```python
from build123d import *

# Parameters (mm, degrees)
BOSS_EXTRUDE2_DEPTH = 2
BOSS_EXTRUDE3_DEPTH = 10.9


with BuildPart() as part:
    # Sketch1 → Boss-Extrude2 (new body)
    with BuildSketch(Plane(origin=(0, 0, 0), x_dir=(1, 0, 0), z_dir=(0, 1, 0))):
        with BuildLine():
            Line((0, 28.575), (137.052797764, 28.575))
            ThreePointArc((137.052797764, 28.575), (139.26125033, 14.36329198), (140, 0))
            ThreePointArc((140, 0), (139.26125033, -14.36329198), (137.052797764, -28.575))
            Line((137.052797764, -28.575), (0, -28.575))
            ThreePointArc((0, -28.575), (-28.575, 0), (0, 28.575))
        make_face()
    extrude(amount=-BOSS_EXTRUDE2_DEPTH)

    # Sketch1_14 → Boss-Extrude3 (add)
    with BuildSketch(Plane(origin=(0, 0, 0), x_dir=(1, 0, 0), z_dir=(0, 1, 0))):
        with BuildLine():
            Line((0, 28.575), (137.052797764, 28.575))
            ThreePointArc((137.052797764, 28.575), (139.26125033, 14.36329198), (140, 0))
            ThreePointArc((140, 0), (139.26125033, -14.36329198), (137.052797764, -28.575))
            Line((137.052797764, -28.575), (0, -28.575))
            ThreePointArc((0, -28.575), (-28.575, 0), (0, 28.575))
        make_face()
        with BuildLine():
            Line((0, -26.575), (130.828205579, -26.575))
            ThreePointArc((130.828205579, -26.575), (132.830371988, -13.354485299), (133.5, 0))
            ThreePointArc((133.5, 0), (132.830371988, 13.354485299), (130.828205579, 26.575))
            Line((130.828205579, 26.575), (0, 26.575))
            ThreePointArc((0, 26.575), (-26.575, 0), (0, -26.575))
        make_face(mode=Mode.SUBTRACT)
    extrude(amount=BOSS_EXTRUDE3_DEPTH)


solid = part.part
```
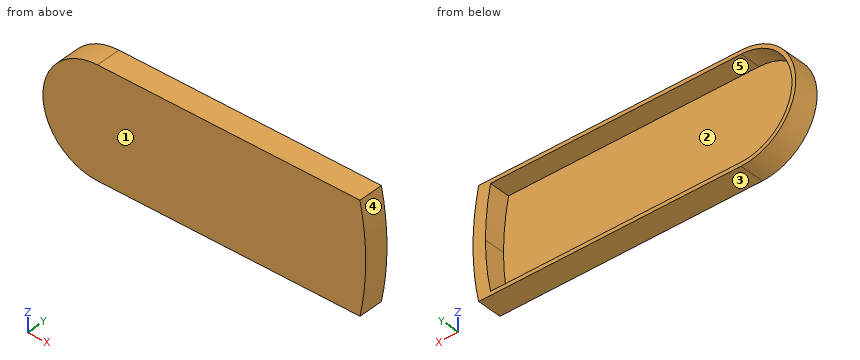
Can you work these out from the model? Positions are in its coordinate system, mm. Face numbers are marked on the shaded views. A direction names the side the tool comes from. Round coordinates to 2 decimals unless told otherwise and drop trailing zeros. Loops run counter-clockwise (first coordinate to the right, second up) from the corner with the lowest first, then second, coordinate; pieces in that order, holes last.
Item 1: Will these pins go through, and if not, where does the flat tip stop? pin 1 Ø6 at (y, z) = (9, 18) entering from +X; pin 2 Ø1.5 at (x, z) = (93.5, 17.5) entering from +Y; pin 3 Ø2 at (y, z) = (1, -8.5) entering from -X.
Item 2: Suppose I cut it at C-C, the plane z = -13. Write out the boundary of the cut face in (x, y), then the cut area to 3 significant figures.
Item 3: Which directions (+Z, -Z, +X, -X, +Y, -Y) give clear straight access to the entire face, cutting with the end or side of a thin tool? Please do the marked faces 1 and 2.
Item 4: Please list where these lines run through material, in increasing order: L1, parallel to Z at x = 91, y = 2 (3 decimals); L2, parallel to X at y = 3.25, z = -0.5; L3, parallel to Y at x = 32, z = 12.5.
Item 5: Suppose I cut it at B-B, the plane x = 70.5. Write out the boundary of the cut face in (y, z) (3 decimals).
Item 6: Suppose I cut it at A-A, the plane y = 7.5. Write out the boundary of the cut face in (x, z) (3 decimals), then the cut area to 3 significant figures.
Item 7: If we mould it in two halves opening along Z, with no side actions, what happens to the marked faces 3, 4 and 5? For each: +Z half, -Z half, draft (parallel to the pull), parting line (faces both ways), or undercut.
Reported:
1. pin 1: stops at x = 139.19
1. pin 2: stops at y = 0
1. pin 3: stops at x = -27.57
2. outline: (-25.45, -2) - (139.4, -2) - (139.4, 10.9) - (132.87, 10.9) - (132.87, 0) - (-23.18, 0) - (-23.18, 10.9) - (-25.45, 10.9) - close
2. area: 426 mm2
3. face 1: +Z, -Z, +X, -X, -Y
3. face 2: +Y
4. L1: z = -28.575 to -26.575, 26.575 to 28.575
4. L2: x = -28.57 to -26.57, 133.5 to 140
4. L3: y = -2 to 0
5. outline: (-2, -28.575) - (10.9, -28.575) - (10.9, -26.575) - (0, -26.575) - (0, 26.575) - (10.9, 26.575) - (10.9, 28.575) - (-2, 28.575) - close
6. outline: (0, -28.575) - (137.053, -28.575) arc R140 ccw to (137.053, 28.575) - (0, 28.575) arc R28.575 ccw to start; hole (0, -26.575) - (130.828, -26.575) arc R133.5 ccw to (130.828, 26.575) - (0, 26.575) arc R26.575 ccw to start
6. area: 1,070 mm2
7. face 3: -Z half
7. face 4: parting line
7. face 5: undercut
